```python
from build123d import *

# Parameters (mm, degrees)
SKETCH1_W           = 3.1
SKETCH1_H           = 45
BOSS_EXTRUDE1_DEPTH = 3
SKETCH3_R           = 1.6
CUT_EXTRUDE2_DEPTH  = 10
CUT_EXTRUDE4_REACH  = 107.547
SKETCH5_R           = 1.65
SKETCH6_R           = 1.65
CUT_EXTRUDE5_DEPTH  = 10
SKETCH8_W           = 30
SKETCH8_H           = 70
CUT_EXTRUDE6_DEPTH  = 10
FILLET1_R           = 5
SKETCH9_R           = 2.1
CUT_EXTRUDE7_DEPTH  = 10


with BuildPart() as part:
    # Sketch1 → Boss-Extrude1 (new body)
    with BuildSketch(Plane(origin=(0, 0, 0), x_dir=(1, 0, 0), z_dir=(0, 1, 0))):
        Polygon((-62.5, -75), (-62.5, -85), (62.5, -85), (62.5, -75), (62.5, -5), (62.5, 85), (-62.5, 85), (-62.5, -5), align=None)
        with Locations((-41.55, -50)):
            Rectangle(SKETCH1_W, SKETCH1_H, mode=Mode.SUBTRACT)
        with Locations((41.55, -50)):
            Rectangle(SKETCH1_W, SKETCH1_H, mode=Mode.SUBTRACT)
    extrude(amount=BOSS_EXTRUDE1_DEPTH)

    # Sketch3 → Cut-Extrude2 (cut)
    with BuildSketch(Plane(origin=(0, 3, 0), x_dir=(1, 0, 0), z_dir=(0, 1, 0))):
        with Locations(Location((-24.15, 46.1, 0), (0, 0, 270))):
            Circle(SKETCH3_R)
        with Locations(Location((24.15, 44.7, 0), (0, 0, 270))):
            Circle(SKETCH3_R)
        with Locations(Location((-18.95, -6.1, 0), (0, 0, 270))):
            Circle(SKETCH3_R)
        with Locations(Location((9, -6.1, 0), (0, 0, 270))):
            Circle(SKETCH3_R)
    extrude(amount=-CUT_EXTRUDE2_DEPTH, mode=Mode.SUBTRACT)

    # Sketch5 → Cut-Extrude4 (cut, up to next)
    with BuildSketch(Plane.XZ, mode=Mode.PRIVATE) as cut_extrude4_sk1:
        with Locations(Location((11.5, -77.5, 0), (0, 0, 270))):
            Circle(SKETCH5_R)
    cut_extrude4_tool1 = extrude(cut_extrude4_sk1.sketch, amount=-CUT_EXTRUDE4_REACH, mode=Mode.PRIVATE) & part.part
    # Sketch5 → Cut-Extrude4 (cut, up to next)
    with BuildSketch(Plane.XZ, mode=Mode.PRIVATE) as cut_extrude4_sk2:
        with Locations(Location((-11.5, -77.5, 0), (0, 0, 270))):
            Circle(SKETCH5_R)
    cut_extrude4_tool2 = extrude(cut_extrude4_sk2.sketch, amount=-CUT_EXTRUDE4_REACH, mode=Mode.PRIVATE) & part.part
    add(cut_extrude4_tool1.solids().sort_by_distance((11.5, 0, -77.5))[0], mode=Mode.SUBTRACT)
    add(cut_extrude4_tool2.solids().sort_by_distance((-11.5, 0, -77.5))[0], mode=Mode.SUBTRACT)

    # Sketch6 → Cut-Extrude5 (cut)
    with BuildSketch(Plane(origin=(0, 3, 0), x_dir=(1, 0, 0), z_dir=(0, 1, 0))):
        with Locations(Location((21, -50, 0), (0, 0, 270))):
            Circle(SKETCH6_R)
        with Locations(Location((-21, -50, 0), (0, 0, 270))):
            Circle(SKETCH6_R)
    extrude(amount=-CUT_EXTRUDE5_DEPTH, mode=Mode.SUBTRACT)

    # Sketch8 → Cut-Extrude6 (cut)
    with BuildSketch(Plane(origin=(0, 3, 0), x_dir=(1, 0, 0), z_dir=(0, 1, 0))):
        with Locations((-47.5, 17.5)):
            Rectangle(SKETCH8_W, SKETCH8_H)
        Polygon((-21, 52.5), (-21, 85), (-62.5, 85), (-62.5, 52.5), (-32.5, 52.5), align=None)
        Polygon((32.5, 52.5), (62.5, 52.5), (62.5, 85), (21, 85), (21, 52.5), align=None)
        with Locations((47.5, 17.5)):
            Rectangle(SKETCH8_W, SKETCH8_H)
    extrude(amount=-CUT_EXTRUDE6_DEPTH, mode=Mode.SUBTRACT)

    # Fillet1
    fillet1_edges = [part.edges().sort_by_distance(p)[0] for p in [
        (21, 1.5, -52.5),
        (21, 1.5, -85),
        (62.5, 1.5, 17.5),
        (32.5, 1.5, 17.5),
        (32.5, 1.5, -52.5),
        (-32.5, 1.5, -52.5),
        (-32.5, 1.5, 17.5),
        (-62.5, 1.5, 17.5),
        (-21, 1.5, -85),
        (-21, 1.5, -52.5),
    ]]
    fillet(fillet1_edges, radius=FILLET1_R)

    # Sketch9 → Cut-Extrude7 (cut)
    with BuildSketch(Plane(origin=(0, 3, 0), x_dir=(1, 0, 0), z_dir=(0, 1, 0))):
        with Locations(Location((19.5, 25, 0), (0, 0, 270))):
            Circle(SKETCH9_R)
        with Locations(Location((-19.5, 25, 0), (0, 0, 270))):
            Circle(SKETCH9_R)
    extrude(amount=-CUT_EXTRUDE7_DEPTH, mode=Mode.SUBTRACT)


solid = part.part
```
Input: part model. Units: mm. Frame: model coordinates. Coordinates: 2 decimals unless noted, no trailing zeros. Write each loop counter-clockwise with the first axis right and the second up, starting at its lowest first coordinate (ties: lowest second). Pieces come first, ordered by that corner, then holes. Notation, with made-up numbers: (38, 56) -> (76, 56) arc R23 cw to (76, 95) -> close; hole circle Ø11 at (-9.75, 43). An arc over 180 degrees is marked (long way). Answer as a JSON object with one key per item and string values.
1. Section B-B on y = 1.2. Count the separate pieces of the cut face and the enclosed holes in it, then the cut area to 3 significant figures.
Result set:
{"separate pieces": "1", "enclosed holes": "12", "area": "14,000 mm2"}
2. Section A-A on z = 61.5. Return the cut outline in (x, y).
Result set:
{"outline": "(-62.5, 0) -> (-43.1, 0) -> (-43.1, 3) -> (-62.5, 3) -> close; (-40, 0) -> (40, 0) -> (40, 3) -> (-40, 3) -> close; (43.1, 0) -> (62.5, 0) -> (62.5, 3) -> (43.1, 3) -> close"}
3. Section C-C on x = -51. Return the cut outline in (y, z), then the cut area to 4 significant figures.
Result set:
{"outline": "(0, 17.5) -> (3, 17.5) -> (3, 85) -> (0, 85) -> close", "area": "202.5 mm2"}
4. First-contact query: P1, Ø1.5, axis at x = 41.5, y = 1.5, coming from the -Z side; P2, Ø0.8, axis at x = 27, y = 1, coming from the -Z side; P3, Ø1.5, axis at x = 23.5, y = 2.5, coming from the -Z side; P4, Ø8, axis at x = -22.5, z = -47.5, coming from the -Y side. Flat tips, straight axial feed; report the tip coordinate or a pass-through.
Result set:
{"P1": "stops at z = 17.5", "P2": "stops at z = -52.5", "P3": "stops at z = -53.7", "P4": "stops at y = 0"}
5. Mould query, pull axis X, two halves, no side actions, for faces 1 (the face through (22.39, 1.52, 50.89)), 2 (the face through (-31.07, 1.48, -51)), 3 (the face through (21.27, 1.52, -23.87)), 4 (the face through (31, 1.48, -51.07)). Classes: released by +X, released by -X, zero draft, split by the parting line, or undercut.
Result set:
{"face 1": "undercut", "face 2": "released by -X", "face 3": "undercut", "face 4": "released by +X"}
6. Material intervals for line 1 (X direction, y = 0.7, z = 6.1); line 2 (X direction, y = 2.4, z = -25); line 3 (X direction, y = 0.75, z = 50), sorted ascending. Write a range as from..to.
Result set:
{"line 1": "x = -32.5..-20.55, -17.35..7.4, 10.6..32.5", "line 2": "x = -32.5..-21.6, -17.4..17.4, 21.6..32.5", "line 3": "x = -62.5..-43.1, -40..-22.65, -19.35..19.35, 22.65..40, 43.1..62.5"}
